from build123d import *

# Parameters (mm, degrees)
SKETCH1_W           = 50
SKETCH1_H           = 60
BOSS_EXTRUDE1_DEPTH = 5
SKETCH2_W           = 20.5
SKETCH2_H           = 40.5
CUT_EXTRUDE1_DEPTH  = 5
SKETCH3_R           = 1.8
CUT_EXTRUDE2_DEPTH  = 5
SKETCH4_R           = 2.5
CUT_EXTRUDE3_DEPTH  = 5
FILLET1_R           = 10
SKETCH5_W           = 5
SKETCH5_H           = 5
CUT_EXTRUDE4_DEPTH  = 10
FILLET2_R           = 1


with BuildPart() as part:
    # Sketch1 → Boss-Extrude1 (new body)
    with BuildSketch(Plane(origin=(0, 0, 0), x_dir=(1, 0, 0), z_dir=(0, 1, 0))):
        Rectangle(SKETCH1_W, SKETCH1_H)
    extrude(amount=BOSS_EXTRUDE1_DEPTH)

    # Sketch2 → Cut-Extrude1 (cut)
    with BuildSketch(Plane(origin=(0, 5, 0), x_dir=(1, 0, 0), z_dir=(0, 1, 0))):
        with Locations((8, 0)):
            Rectangle(SKETCH2_W, SKETCH2_H)
    extrude(amount=-CUT_EXTRUDE1_DEPTH, mode=Mode.SUBTRACT)

    # Sketch3 → Cut-Extrude2 (cut)
    with BuildSketch(Plane(origin=(0, 5, 0), x_dir=(1, 0, 0), z_dir=(0, 1, 0))):
        with Locations((3, 24.75)):
            Circle(SKETCH3_R)
        with Locations((13, 24.75)):
            Circle(SKETCH3_R)
        with Locations((13, -24.75)):
            Circle(SKETCH3_R)
        with Locations((3, -24.75)):
            Circle(SKETCH3_R)
    extrude(amount=-CUT_EXTRUDE2_DEPTH, mode=Mode.SUBTRACT)

    # Sketch4 → Cut-Extrude3 (cut)
    with BuildSketch(Plane(origin=(0, 5, 0), x_dir=(1, 0, 0), z_dir=(0, 1, 0))):
        with Locations((-17.5, 20)):
            Circle(SKETCH4_R)
        with Locations((-17.5, -20)):
            Circle(SKETCH4_R)
    extrude(amount=-CUT_EXTRUDE3_DEPTH, mode=Mode.SUBTRACT)

    # Fillet1
    fillet1_edges = [part.edges().sort_by_distance(p)[0] for p in [
        (-25, 2.5, -30),
        (25, 2.5, -30),
        (25, 2.5, 30),
        (-25, 2.5, 30),
    ]]
    fillet(fillet1_edges, radius=FILLET1_R)

    # Sketch5 → Cut-Extrude4 (cut)
    with BuildSketch(Plane(origin=(0, 5, 0), x_dir=(1, 0, 0), z_dir=(0, 1, 0))):
        with Locations((8, 20.25)):
            Rectangle(SKETCH5_W, SKETCH5_H)
    cut_extrude4 = extrude(amount=-CUT_EXTRUDE4_DEPTH, mode=Mode.SUBTRACT)

    # Mirror1: Cut-Extrude4 across plane
    add(cut_extrude4.mirror(Plane.XY), mode=Mode.SUBTRACT)

    # Fillet2
    fillet2_edges = [part.edges().sort_by_distance(p)[0] for p in [
        (10.5, 2.5, 20.25),
        (5.5, 2.5, 20.25),
        (10.5, 2.5, 22.75),
        (5.5, 2.5, 22.75),
        (10.5, 2.5, -20.25),
        (5.5, 2.5, -20.25),
        (5.5, 2.5, -22.75),
        (10.5, 2.5, -22.75),
    ]]
    fillet(fillet2_edges, radius=FILLET2_R)


solid = part.part
Design review of the part built by this model. Coordinates are the model's own, in mm. A direction names the side the tool comes from. Give positions to 0.01 mm unless a question says otherwise; leave off trailing zeros. Order: outer loops, then holes, each group sorted by start corner. A loop starts at its lowest first (then second) coordinate and runs counter-clockwise, first axis right, second up. Notation, with made-up numbers: (-31.75, 89.5) - (-3.75, 89.5) arc R19 cw to (-3.75, 111.5) - close; hole circle Ø7 at (21.25, -23.5). An arc over 180 degrees is marked (long way). Write item = value, one per line. Start each with the question number.
Q1. To check wall thickness, follow L1, parallel to Z at x = 13, y = 3.1; L2, parallel to X at y = 1, z = -10.5; L3, parallel to X at y = 3.3, z = -24.75. State the ranges of each line that lie inside material, in increasing order. Write a range as from..to.
Q2. Tool access review of faces 1 (the face through (0, 2, -30)), 2 (the face through (1, 3, 20.25)): name each direction out of +Z, -Z, +X, -X, +Y, -Y from which nothing blocks a thin tool from reaching the whole face with its end or side.
Q3. We need section B-B on x = 3. State the section outline as (y, z) points, plus the area to 3 significant figures.
Q4. Clearance check with flat-ended pins moving along their axes: pin 1 Ø3 at (y, z) = (2.5, 23.5) entering from -X; pin 2 Ø4 at (x, z) = (-17.5, -20) entering from +Y; pin 3 Ø0.6 at (y, z) = (2.5, 21.5) entering from -X; pin 4 Ø0.6 at (y, z) = (2.5, 21.5) entering from +X. State where each tip first meets the part, or that it passes through.
Q5. We need section D-D on z = 24.75. State the section outline as (x, y) points, plus the area to 3 significant figures.
Q6. Mouldability with a two-part tool opening along X and no side actions: class faces 3 (the face through (-22.15, 2.54, 26.99)), 4 (the face through (-19, 3, -22)), 5 (the face through (25, 2, 0)) as released by +X, released by -X, zero draft, split by the parting line, or undercut.
Q7. We need section C-C on y = 3.95. State how many separate pieces and enclosed holes the cut face has, plus the area to 3 significant figures.
Q8. We need section A-A on z = -7. State the section outline as (x, y) points, plus the area to 4 significant figures.
Working result:
q1.L1 = -30..-26.55, -22.95..-20.25, 20.25..22.95, 26.55..30
q1.L2 = -25..-2.25, 18.25..25
q1.L3 = -23.8..1.2, 4.8..11.2, 14.8..23.8
q2.face_1 = -Z, +X, -X, +Y, -Y
q2.face_2 = +Y, -Y
q3.outline = (0, -30) - (5, -30) - (5, -26.55) - (0, -26.55) - close; (0, -22.95) - (5, -22.95) - (5, -20.25) - (0, -20.25) - close; (0, 20.25) - (5, 20.25) - (5, 22.95) - (0, 22.95) - close; (0, 26.55) - (5, 26.55) - (5, 30) - (0, 30) - close
q3.area = 61.5 mm²
q4.pin_1 = -24.8
q4.pin_2 = through
q4.pin_3 = -24.93
q4.pin_4 = 24.93
q5.outline = (-23.8, 0) - (1.2, 0) - (1.2, 5) - (-23.8, 5) - close; (4.8, 0) - (11.2, 0) - (11.2, 5) - (4.8, 5) - close; (14.8, 0) - (23.8, 0) - (23.8, 5) - (14.8, 5) - close
q5.area = 202 mm²
q6.face_3 = released by -X
q6.face_4 = undercut
q6.face_5 = released by +X
q7.separate_pieces = 1
q7.enclosed_holes = 7
q7.area = 1,980 mm²
q8.outline = (-25, 0) - (-2.25, 0) - (-2.25, 5) - (-25, 5) - close; (18.25, 0) - (25, 0) - (25, 5) - (18.25, 5) - close
q8.area = 147.5 mm²
